from build123d import *

# Parameters (mm, degrees)
F0_R     = 3
F0_R_2   = 2.25
F1_DEPTH = 5
F1_TAPER = 20
F2_DEPTH = 3
F3_DEPTH = 25
F4_R     = 1
F5_DEPTH = 25


with BuildPart() as f1:
    # F0 (on Top) → F1 (new body)
    with BuildSketch(Plane.XY):
        with BuildLine():
            Line((4.5, -3.9686269666), (4.5, 3.9686269666))
            ThreePointArc((4.5, 3.9686269666), (-6, 0), (4.5, -3.9686269666))
        make_face()
        Circle(F0_R, mode=Mode.SUBTRACT)
        Circle(F0_R)
        Circle(F0_R_2, mode=Mode.SUBTRACT)
        Circle(F0_R_2)
        with BuildLine():
            ThreePointArc((4.5, -3.9686269666), (5.6124860802, -2.1213203436), (6, 0))
            ThreePointArc((6, 0), (5.6124860802, 2.1213203436), (4.5, 3.9686269666))
            Line((4.5, 3.9686269666), (4.5, -3.9686269666))
        make_face()
    extrude(amount=F1_DEPTH, taper=F1_TAPER)

    # F0 (on Top) → F2 (cut)
    with BuildSketch(Plane.XY):
        Circle(F0_R)
        Circle(F0_R_2, mode=Mode.SUBTRACT)
    extrude(amount=F2_DEPTH, mode=Mode.SUBTRACT)

    # F0 (on Top) → F3 (cut)
    with BuildSketch(Plane.XY):
        Circle(F0_R_2)
    extrude(amount=F3_DEPTH, mode=Mode.SUBTRACT)

    # F4
    f4_edges = [f1.edges().sort_by_distance(p)[0] for p in [
        (-3.135112, 2.764909, 5),
    ]]
    fillet(f4_edges, radius=F4_R)

    # F0 (on Top) → F5 (cut)
    with BuildSketch(Plane.XY):
        with BuildLine():
            ThreePointArc((4.5, -3.9686269666), (5.6124860802, -2.1213203436), (6, 0))
            ThreePointArc((6, 0), (5.6124860802, 2.1213203436), (4.5, 3.9686269666))
            Line((4.5, 3.9686269666), (4.5, -3.9686269666))
        make_face()
    extrude(amount=F5_DEPTH, mode=Mode.SUBTRACT)


solid = f1.part
For this review, take the finished solid that the model builds, in its own axes (mm). A direction names the side the tool comes from. Round coordinates to 2 decimals unless told otherwise and drop trailing zeros. Order: outer loops, then holes, each group sorted by start corner. A loop starts at its lowest first (then second) coordinate and runs counter-clockwise, first axis right, second up. Notation, with made-up numbers: (56, -19.75) -> (76, -19.75) arc R9 cw to (76, -14.75) -> close; hole circle Ø11 at (-37.75, -1.75). An arc over 180 degrees is marked (long way). Write item = value, one per line. Start each with the question number.
1) Insertion check: pin 1 (3 mm diameter, centred on x = -0.5, z = 4.5, fed in from -Y); pin 2 (1 mm diameter, centred on y = 0.5, z = 1, fed in from -X); pin 3 (1 mm diameter, centred on x = -1.5, z = 4, fed in from -Y); pin 4 (1.5 mm diameter, centred on x = 0.5, y = -2.5, fed in from -Z). Each pin has a flat end and moves straight along its axis. Give the tip position at first contact, or say it passes through.
2) To check wall thickness, follow line 1 (X direction, y = -2, z = 0.8); line 2 (Y direction, x = 0, z = 2.3); line 3 (X direction, y = 1.5, z = 1.6). State the ranges of each line that lie inside material, in increasing order. Write a range as from..to.
3) Take a section at A-A on z = 3.3. State the section outline as (x, y) points.
4) Take a section at C-C on z = 4.7. State the section outline as (x, y) points, plus the area to 3 significant figures.
5) Tool access review of faces 1 (the face through (-3, 0, 1)), 2 (the face through (-3.2, 0.1, 0)): name each direction out of +Z, -Z, +X, -X, +Y, -Y from which nothing blocks a thin tool from reaching the whole face with its end or side.
6) Take a section at B-B on z = 0.9. State the section outline as (x, y) points, plus the area to 3 significant figures.
7) The part is to be moulded in two halves that separate along X. For faces 3 (the face through (-0.29, 2.23, 3.99)), 4 (the face through (4.5, 0, 2)), 5 (the face through (2.3, -0.7, 5)), say which applies: +X half, -X half, draft (parallel to the pull), parting line (faces both ways), or undercut.
Verdict:
q1.pin_1 = -4.89
q1.pin_2 = -5.8
q1.pin_3 = -4.53
q1.pin_4 = 0
q2.line_1 = -5.35..-2.24, 2.24..4.5
q2.line_2 = -5.16..-3, 3..5.16
q2.line_3 = -5.21..-2.6, 2.6..4.5
q3.outline = (4.5, -1.67) -> (4.5, 1.67) arc R4.8 ccw (long way) to start; hole circle Ø4.5 at (0, 0)
q4.outline = circle Ø8.39 at (0, 0); hole circle Ø4.5 at (0, 0)
q4.area = 39.4 mm2
q5.face_1 = -Z
q5.face_2 = -Z, +X, -X, +Y, -Y
q6.outline = (4.5, -3.45) -> (4.5, 3.45) arc R5.67 ccw (long way) to start; hole circle Ø6 at (0, 0)
q6.area = 67.3 mm2
q7.face_3 = undercut
q7.face_4 = +X half
q7.face_5 = draft
